from build123d import *

# Parameters (mm, degrees)
F1_DEPTH = 20
F2_W     = 100
F2_H     = 100
F3_DEPTH = 21
F5_DEPTH = 130


with BuildPart() as f1:
    # F0 (on Front) → F1 (new body)
    with BuildSketch(Plane.XZ):
        Polygon((-31.066017178, -75), (31.066017178, -75), (53.033008589, -53.033008589), (-53.033008589, -53.033008589), align=None)
        Polygon((54.3077377365, 51.7582794414), (53.033008589, -53.033008589), (75, -31.066017178), (75, 31.066017178), align=None)
        Polygon((-53.033008589, -53.033008589), (53.033008589, -53.033008589), (54.3077377365, 51.7582794414), (-53.033008589, 53.033008589), align=None)
        Polygon((-75, -31.066017178), (-53.033008589, -53.033008589), (-53.033008589, 53.033008589), (-75, 31.066017178), align=None)
        Polygon((-53.033008589, 53.033008589), (54.3077377365, 51.7582794414), (31.066017178, 75), (-31.066017178, 75), align=None)
    extrude(amount=-F1_DEPTH)

    # F2 (on face) → F3 (join)
    with BuildSketch(Plane.XZ):
        Rectangle(F2_W, F2_H)
    extrude(amount=-F3_DEPTH)

    # F4 (on face) → F5 (join)
    with BuildSketch(Plane.XZ):
        Polygon((0, 70.7106781187), (-35.3553390593, 35.3553390593), (-70.7106781187, 0), (0, -70.7106781187), (70.7106781187, 0), align=None)
    extrude(amount=F5_DEPTH)


solid = f1.part
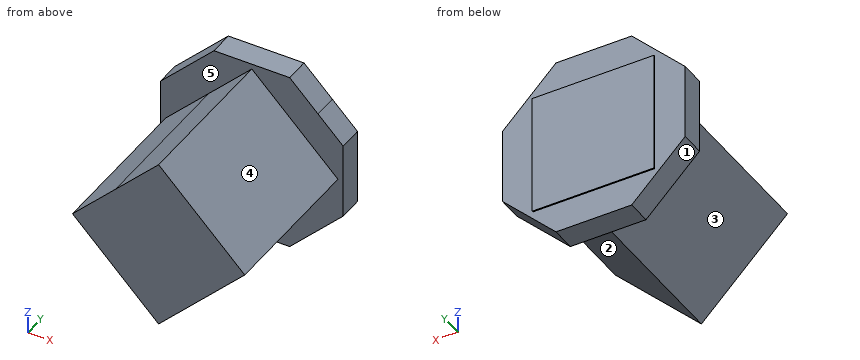
Design review of the part built by this model. Coordinates are the model's own, in mm. Face numbers are marked on the shaded views. A direction names the side the tool comes from. Round coordinates to 2 decimals unless told otherwise and drop trailing zeros. Write each loop counter-clockwise with the first axis right and the second up, starting at its lowest first coordinate (ties: lowest second). Pieces come first, ordered by that corner, then holes. Notation, with made-up numbers: (28, 36.25) - (58, 36.25) arc R21 cw to (58, 63.25) - close; hole circle Ø4 at (43, -36.75). An arc over 180 degrees is marked (long way). Return JSON: item names as keys, results as strings. Group by question number.
Item 1: We need section B-B on x = 58. Write out the cut boundary in (y, z), and give its area (3 significant figures).
Item 2: We need section C-C on z = -20. Write out the cut boundary in (x, y).
Item 3: For probe 1 along Y at (x, z) = (-41, -38.5); probe 2 along Y at (x, z) = (52, -20.5); probe 3 along Z at (x, y) = (-40, -41), list the stretches that pass through material, from the lowest coordinate up. Write a range as [from, to].
Item 4: We need section D-D on x = -39. Write out the cut boundary in (y, z).
Item 5: We need section A-A on y = -119. Write out the cut boundary in (x, z).
Item 6: Machinability: for the marked faces 1, 2, 3, 4 and 5, which of the approach directions +Z, -Z, +X, -X, +Y, -Y give a long, thin tool a straight path to every point of the face, cutting with its end or side? Answer none if there is none.
Item 7: Insertion check: P1, Ø3, axis at x = -59, y = -102.5, coming from the -Z side; P2, Ø8, axis at x = 16.5, y = -45, coming from the +Z side; P3, Ø5, axis at y = -80, z = -32, coming from the -X side. Each pin has a flat end and moves straight along its axis. Give the tip position at first contact, or say it passes through.
Model answer:
{
 "1": {"outline": "(-130, -12.71) - (0, -12.71) - (0, -48.07) - (20, -48.07) - (20, 48.07) - (0, 48.07) - (0, 12.71) - (-130, 12.71) - close", "area": "5,230 mm²"},
 "2": {"outline": "(-75, 0) - (-50.71, 0) - (-50.71, -130) - (50.71, -130) - (50.71, 0) - (75, 0) - (75, 20) - (50, 20) - (50, 21) - (-50, 21) - (-50, 20) - (-75, 20) - close"},
 "3": {"probe 1": "y = [0, 21]", "probe 2": "y = [0, 20]", "probe 3": "z = [-30.71, 30.71]"},
 "4": {"outline": "(-130, -31.71) - (0, -31.71) - (0, -67.07) - (20, -67.07) - (20, -50) - (21, -50) - (21, 50) - (20, 50) - (20, 67.07) - (0, 67.07) - (0, 31.71) - (-130, 31.71) - close"},
 "5": {"outline": "(-70.71, 0) - (0, -70.71) - (70.71, 0) - (0, 70.71) - close"},
 "6": {"face 1": "-Z, -X, +Y, -Y", "face 2": "-Z, +X, -Y", "face 3": "-Z, -X, -Y", "face 4": "+Z, +X, -Y", "face 5": "-Y"},
 "7": {"P1": "stops at z = -13.21", "P2": "stops at z = 58.21", "P3": "stops at x = -41.21"}
}
